The figure shows three views and two pictorial views of one solid part (mm, origin at its lowest corner). Answer the questions. Coordinates: 2 decimals unless noted, no trailing zeros. Loops run counter-clockwise (first coordinate to the right, second up) from the corner with the lowest first, then second, coordinate; pieces in that order, holes last.
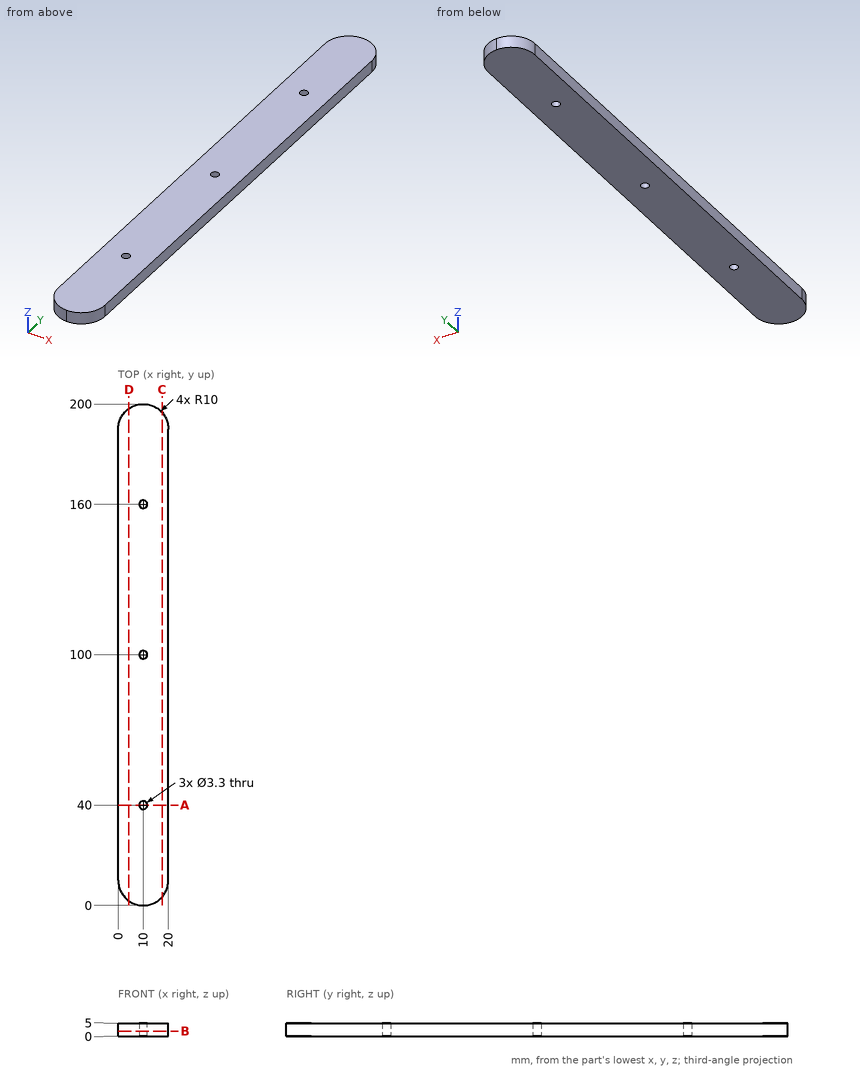
1. Each of these flat-tipped pins is pushed along its axis until it touches: P1, Ø2, axis at x = 16, z = 4, coming from the -Y side; P2, Ø2, axis at x = 10, y = 160, coming from the -Z side. Where does it stop, or does it pass through?
2. A cutting plane is placed at C-C, the plane x = 17.5. Give the vertices of the cut face in (y, z).
3. A cutting plane is placed at D-D, the plane x = 4.25. Give the vertices of the cut face in (y, z).
4. Straight lines are drawn through the part: probe 1 along Y at (x, z) = (10, 2.05); probe 2 along Y at (x, z) = (9, 0.3); probe 3 along X at (y, z) = (100, 3.8). For each, find the intervals that lie inside material, in ascending order.
5. A cutting plane is placed at A-A, the plane y = 40. Give the vertices of the cut face in (x, z), then the cut area to 3 significant figures.
6. A cutting plane is placed at B-B, the plane z = 1.9. Count the separate pieces of the cut face and the enclosed holes in it, then the cut area to 3 significant figures.
Answers below:
1. P1: stops at y = 1.34
1. P2: passes through
2. outline: (3.39, 0) - (196.61, 0) - (196.61, 5) - (3.39, 5) - close
3. outline: (1.82, 0) - (198.18, 0) - (198.18, 5) - (1.82, 5) - close
4. probe 1: y = 0 to 38.35, 41.65 to 98.35, 101.65 to 158.35, 161.65 to 200
4. probe 2: y = 0.05 to 38.69, 41.31 to 98.69, 101.31 to 158.69, 161.31 to 199.95
4. probe 3: x = 0 to 8.35, 11.65 to 20
5. outline: (0, 0) - (8.35, 0) - (8.35, 5) - (0, 5) - close; (11.65, 0) - (20, 0) - (20, 5) - (11.65, 5) - close
5. area: 83.5 mm2
6. separate pieces: 1
6. enclosed holes: 3
6. area: 3,890 mm2
